Drawing for the job (mm, zero at the part's lowest x, y, z). Coordinates: 2 decimals unless noted, no trailing zeros. Write each loop counter-clockwise with the first axis right and the second up, starting at its lowest first coordinate (ties: lowest second). Pieces come first, ordered by that corner, then holes. Notation, with made-up numbers: (-22, 40) -> (13, 40) arc R30 cw to (13, 76) -> close; hole circle Ø8 at (89.5, -1.75). An arc over 180 degrees is marked (long way). Write each question's results on one line, items separated by ' | '. Start each with the question number.
Q1. Saw through at C-C on y = 3. Give the cut face in (x, z), and give its area (3 significant figures).
Q2. Saw through at A-A on x = 46.75. Give the cut face in (y, z), and give its area (3 significant figures).
Q3. Saw through at B-B on z = 1.25. Count the separate pieces of the cut face and the enclosed holes in it, and give its area (3 significant figures).
Q4. Drill centre lines: line 1 (Y direction, x = 31.25, z = 0.65); line 2 (Y direction, x = 46.75, z = 0.6); line 3 (X direction, y = 2.2, z = 1). Where is each one in solid material? Low to high.
Q5. Drop a flat-ended pin along its axis: pin 1 Ø3 at (x, y) = (46.75, 3) entering from -Z. Give the stop position or say it passes through.
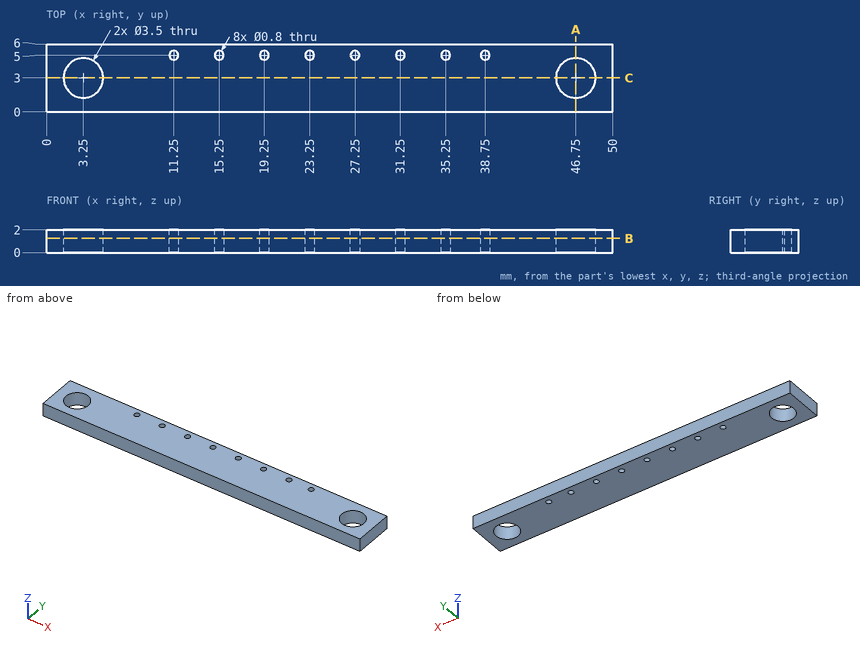
Returned:
1) outline: (0, 0) -> (1.5, 0) -> (1.5, 2) -> (0, 2) -> close; (5, 0) -> (45, 0) -> (45, 2) -> (5, 2) -> close; (48.5, 0) -> (50, 0) -> (50, 2) -> (48.5, 2) -> close | area: 86.0 mm2
2) outline: (0, 0) -> (1.25, 0) -> (1.25, 2) -> (0, 2) -> close; (4.75, 0) -> (6, 0) -> (6, 2) -> (4.75, 2) -> close | area: 5.00 mm2
3) separate pieces: 1 | enclosed holes: 10 | area: 277 mm2
4) line 1: y = 0 to 4.6, 5.4 to 6 | line 2: y = 0 to 1.25, 4.75 to 6 | line 3: x = 0 to 1.69, 4.81 to 45.19, 48.31 to 50
5) pin 1: passes through
